Could you check a few things on this drawing? It's one solid part, dimensions in mm from its lowest x, y, z. A direction names the side the tool comes from. Coordinates: 2 decimals unless noted, no trailing zeros. Order: outer loops, then holes, each group sorted by start corner. A loop starts at its lowest first (then second) coordinate and runs counter-clockwise, first axis right, second up. Notation, with made-up numbers: (28, 35.5) -> (46, 35.5) arc R26 cw to (46, 58.5) -> close; hole circle Ø10 at (80.25, 8). An arc over 180 degrees is marked (long way). Answer as CSV lines item,"result".
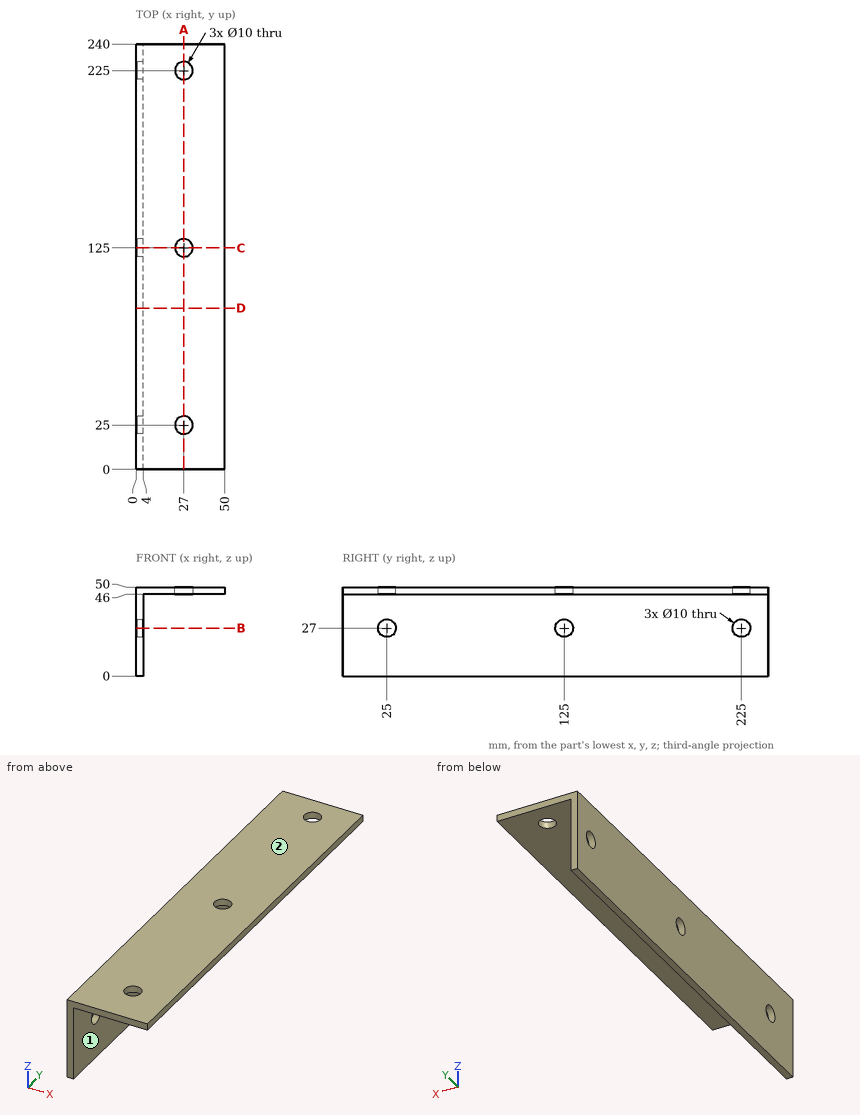
Q1. Imagine slicing it at D-D (y = 91). List the corners of the cut face in (x, z) for me, and give its area (3 significant figures).
Solution:
outline,"(0, 0) -> (4, 0) -> (4, 46) -> (50, 46) -> (50, 50) -> (0, 50) -> close"
area,"384 mm2"
Q2. Which directions (+Z, -Z, +X, -X, +Y, -Y) give clear straight access to the entire face, cutting with the end or side of a thin tool? Please do the marked faces 1 and 2.
Solution:
face 1,"-Z, +X, +Y, -Y"
face 2,"+Z, +X, -X, +Y, -Y"
Q3. Imagine slicing it at B-B (z = 27). List the corners of the cut face in (x, y) for me.
Solution:
outline,"(0, 0) -> (4, 0) -> (4, 20) -> (0, 20) -> close; (0, 30) -> (4, 30) -> (4, 120) -> (0, 120) -> close; (0, 130) -> (4, 130) -> (4, 220) -> (0, 220) -> close; (0, 230) -> (4, 230) -> (4, 240) -> (0, 240) -> close"
Q4. Imagine slicing it at A-A (x = 27). List the corners of the cut face in (y, z) for me.
Solution:
outline,"(0, 46) -> (20, 46) -> (20, 50) -> (0, 50) -> close; (30, 46) -> (120, 46) -> (120, 50) -> (30, 50) -> close; (130, 46) -> (220, 46) -> (220, 50) -> (130, 50) -> close; (230, 46) -> (240, 46) -> (240, 50) -> (230, 50) -> close"
Q5. Imagine slicing it at C-C (y = 125). List the corners of the cut face in (x, z) for me, and give its area (3 significant figures).
Solution:
outline,"(0, 0) -> (4, 0) -> (4, 22) -> (0, 22) -> close; (0, 32) -> (4, 32) -> (4, 46) -> (22, 46) -> (22, 50) -> (0, 50) -> close; (32, 46) -> (50, 46) -> (50, 50) -> (32, 50) -> close"
area,"304 mm2"
Q6. If I drill on line 1 (Y direction, x = 1.8, z = 27); line 2 (Z direction, x = 6, y = 56); line 3 (X direction, y = 212, z = 16), over which ranges is the centre line in solid material (lowest first)?
Solution:
line 1,"0 to 20, 30 to 120, 130 to 220, 230 to 240"
line 2,"46 to 50"
line 3,"0 to 4"
Q7. For P1, Ø23, axis at y = 173, z = 14.5, coming from the +X side; P2, Ø16, axis at x = 27, y = 125, coming from the +Z side; P3, Ø14, axis at x = 16.5, y = 151.5, coming from the -Z side; P4, Ø8, axis at y = 25, z = 27, coming from the -X side, each with a flat end and sliding along its axis, tell me the tip position at first contact or that it passes through.
Solution:
P1,"x = 4"
P2,"z = 50"
P3,"z = 46"
P4,"through"
